Geometry: final body of the model. Coordinates: model frame, mm. A direction names the side the tool comes from. Round coordinates to 2 decimals unless told otherwise and drop trailing zeros. Loops run counter-clockwise (first coordinate to the right, second up) from the corner with the lowest first, then second, coordinate; pieces in that order, holes last. Notation, with made-up numbers: M 45.25,3 L 69.25,3 A17 ccw 69.25,11 Z; hole C 85,68 d10. An arc over 180 degrees is marked long. Answer as a JSON object with one key per item and string values.
from build123d import *

# Parameters (mm, degrees)
SKETCH2_W             = 10
SKETCH2_H             = 101.6
BOSS_EXTRUDE1_DEPTH   = 80
BOSS_EXTRUDE1_2_DEPTH = 80
SKETCH2_3_W           = 10
SKETCH2_3_H           = 101.6
SKETCH2_3_W_2         = 80
BOSS_EXTRUDE2_DEPTH   = 5
SKETCH3_R             = 14.2875
CUT_EXTRUDE1_DEPTH    = 117
SKETCH4_W             = 25.345740838
SKETCH4_H             = 80
CUT_EXTRUDE2_DEPTH    = 119
FILLET3_R             = 10
FILLET2_R             = 10
SKETCH7_R             = 1.6
CUT_EXTRUDE4_DEPTH    = 21
BOSS_EXTRUDE3_START   = 80
SKETCH8_R             = 14.2875
SKETCH8_R_2           = 7.62
BOSS_EXTRUDE3_DEPTH   = 3
SKETCH9_R             = 2.1
CUT_EXTRUDE5_DEPTH    = 5
CUT_EXTRUDE6_DEPTH    = 10
SKETCH10_R            = 2.54
CUT_EXTRUDE7_DEPTH    = 10
FILLET4_R             = 25


with BuildPart() as part:
    # Sketch2 → Boss-Extrude1 (new body)
    with BuildSketch(Plane(origin=(0, 0, 0), x_dir=(1, 0, 0), z_dir=(0, 1, 0))):
        with Locations((-45, 0)):
            Rectangle(SKETCH2_W, SKETCH2_H)
    extrude(amount=BOSS_EXTRUDE1_DEPTH)



with BuildPart() as body_2:
    # Sketch2 → Boss-Extrude1 2 (new body)
    with BuildSketch(Plane(origin=(0, 0, 0), x_dir=(1, 0, 0), z_dir=(0, 1, 0))):
        with Locations((45, 0)):
            Rectangle(SKETCH2_W, SKETCH2_H)
    extrude(amount=BOSS_EXTRUDE1_2_DEPTH)


with BuildPart() as part_1:
    add(part.part)

    add(body_2.part)  # Boss-Extrude2 merges body 2
    # Sketch2<3> → Boss-Extrude2 (add)
    with BuildSketch(Plane(origin=(0, 0, 0), x_dir=(1, 0, 0), z_dir=(0, 1, 0))):
        with Locations((45, 0)):
            Rectangle(SKETCH2_3_W, SKETCH2_3_H)
        Rectangle(SKETCH2_3_W_2, SKETCH2_3_H)
        with Locations((-45, 0)):
            Rectangle(SKETCH2_3_W, SKETCH2_3_H)
    extrude(amount=-BOSS_EXTRUDE2_DEPTH)

    # Sketch3 → Cut-Extrude1 (cut)
    with BuildSketch(Plane.ZY.offset(50)):
        with Locations((0, 50)):
            Circle(SKETCH3_R)
    extrude(amount=-CUT_EXTRUDE1_DEPTH, mode=Mode.SUBTRACT)

    # Sketch4 → Cut-Extrude2 (cut)
    with BuildSketch(Plane(origin=(50, 0, 0), x_dir=(0, 0, -1), z_dir=(1, 0, 0))):
        with Locations((-38.127129581, 40)):
            Rectangle(SKETCH4_W, SKETCH4_H)
        with Locations((38.127129581, 40)):
            Rectangle(SKETCH4_W, SKETCH4_H)
    extrude(amount=-CUT_EXTRUDE2_DEPTH, mode=Mode.SUBTRACT)

    # Fillet3
    fillet3_edges = [part_1.edges().sort_by_distance(p)[0] for p in [
        (45, 80, -25.454259162),
        (45, 80, 25.454259162),
        (40, 0, 0),
        (-40, 0, 0),
        (-45, 0, 25.454259162),
        (45, 0, 25.454259162),
        (-45, 0, -25.454259162),
        (45, 0, -25.454259162),
    ]]
    fillet(fillet3_edges, radius=FILLET3_R)

    # Fillet2
    fillet2_edges = [part_1.edges().sort_by_distance(p)[0] for p in [
        (50, -2.5, -50.8),
        (50, -2.5, 50.8),
        (-50, -2.5, 50.8),
        (-50, -2.5, -50.8),
    ]]
    fillet(fillet2_edges, radius=FILLET2_R)

    # Sketch7 → Cut-Extrude4 (cut)
    with BuildSketch(Plane(origin=(50, 0, 0), x_dir=(0, 0, -1), z_dir=(1, 0, 0))):
        with Locations((-15.5, 65.5)):
            Circle(SKETCH7_R)
        with Locations((15.5, 65.5)):
            Circle(SKETCH7_R)
        with Locations((15.5, 34.5)):
            Circle(SKETCH7_R)
        with Locations((-15.5, 34.5)):
            Circle(SKETCH7_R)
    extrude(amount=-CUT_EXTRUDE4_DEPTH, mode=Mode.SUBTRACT)

    # Sketch8 → Boss-Extrude3 (add)
    with BuildSketch(Plane.ZY.offset(-40).offset(BOSS_EXTRUDE3_START)):
        with Locations((0, 50)):
            Circle(SKETCH8_R)
        with Locations((0, 50)):
            Circle(SKETCH8_R_2, mode=Mode.SUBTRACT)
    extrude(amount=BOSS_EXTRUDE3_DEPTH)

    # Sketch9 → Cut-Extrude5 (cut)
    with BuildSketch(Plane.XZ.offset(5)):
        with Locations((-40.66, 40.66)):
            Circle(SKETCH9_R)
        with Locations((40.66, 40.66)):
            Circle(SKETCH9_R)
        with Locations((-40.66, -40.66)):
            Circle(SKETCH9_R)
        with Locations((40.66, -40.66)):
            Circle(SKETCH9_R)
    extrude(amount=-CUT_EXTRUDE5_DEPTH, mode=Mode.SUBTRACT)

    # Sketch5 → Cut-Extrude6 (cut)
    with BuildSketch(Plane(origin=(0, 0, 0), x_dir=(1, 0, 0), z_dir=(0, 1, 0))):
        with BuildLine():
            Line((-1.917657947, 2.032), (1.917657947, 2.032))
            ThreePointArc((1.917657947, 2.032), (0, -2.794), (-1.917657947, 2.032))
        make_face()
    extrude(amount=-CUT_EXTRUDE6_DEPTH, mode=Mode.SUBTRACT)

    # Sketch10 → Cut-Extrude7 (cut)
    with BuildSketch(Plane(origin=(0, 0, 0), x_dir=(1, 0, 0), z_dir=(0, 1, 0))):
        with Locations((0, 9.099794366)):
            Circle(SKETCH10_R)
    extrude(amount=-CUT_EXTRUDE7_DEPTH, mode=Mode.SUBTRACT)

    # Fillet4
    fillet4_edges = [part_1.edges().sort_by_distance(p)[0] for p in [
        (-45, 80, 25.454259162),
        (-45, 80, -25.454259162),
    ]]
    fillet(fillet4_edges, radius=FILLET4_R)


solid = part_1.part
1) Section query B-B (y = 15). Return the cut outline in (x, z).
Results:
{"outline": "M -50,-25.45 L -40,-25.45 L -40,25.45 L -50,25.45 Z; M 40,-25.45 L 50,-25.45 L 50,25.45 L 40,25.45 Z"}
2) Section query D-D (z = -30.5). Return the cut outline in (x, y), and give its area (3 significant figures).
Results:
{"outline": "M -50,-5 L 50,-5 L 50,1.31 L 34.95,1.31 A10 cw 30,0 L -30,0 A10 cw -34.95,1.31 L -50,1.31 Z", "area": "544 mm2"}
3) Section query A-A (y = 50). Return the cut outline in (x, z).
Results:
{"outline": "M -50,-25.45 L -40,-25.45 L -40,-7.62 L -43,-7.62 L -43,-14.29 L -50,-14.29 Z; M -50,14.29 L -43,14.29 L -43,7.62 L -40,7.62 L -40,25.45 L -50,25.45 Z; M 40,-25.45 L 50,-25.45 L 50,-14.29 L 40,-14.29 Z; M 40,14.29 L 50,14.29 L 50,25.45 L 40,25.45 Z"}
4) Section query C-C (x = -37). Return the cut outline in (y, z), and give its area (3 significant figures).
Results:
{"outline": "M -5,-50.8 L 0,-50.8 L 0,-35.45 A10 cw 2.86,-28.45 L 2.86,28.45 A10 cw 0,35.45 L 0,50.8 L -5,50.8 Z", "area": "683 mm2"}
5) Ray query, line 1 (Y direction, x = 45.75, z = 15.5); line 2 (X direction, y = 17, z = 8.5); line 3 (Y direction, x = -47, z = 0). Return the intervals inside material, ascending.
Results:
{"line 1": "-5 to 32.9, 36.1 to 63.9, 67.1 to 80", "line 2": "-50 to -40, 40 to 50", "line 3": "-5 to 35.71, 64.29 to 80"}
6) Reachability of faces 1 (the flat face through (40, 36.7, 6)), 2 (the cylindrical face through (-46.549, 36.052, -3.097)), 3 (the flat face through (-45, 32, -25.454)) from +Z, -Z, +X, -X, +Y, -Y: full face, straight path, thin tool, end or side. Return the list, or none.
Results:
{"face 1": "+Z, -Z, +Y", "face 2": "-X", "face 3": "-Z, +X, -X, +Y"}
7) Pull-direction query (Y, two-part tool) for faces 4 (the flat face through (-43, 44, 6)), 5 (the cylindrical face through (-42.36, 1.87, 29.63)), 6 (the flat face through (-1, -2, 50.8)); classes: +Y half, -Y half, draft (parallel to the pull), parting line (faces both ways), or undercut.
Results:
{"face 4": "undercut", "face 5": "+Y half", "face 6": "draft"}
8) Pin query (flat end, axial travel): P1, Ø4, axis at x = -32, z = 2, coming from the +Y side; P2, Ø6.5, axis at x = 0, z = 0, coming from the +Y side; P3, Ø3, axis at y = 34.5, z = -15.5, coming from the +X side; P4, Ø3.5, axis at x = -40.66, z = -40.66, coming from the +Y side. Return the tip coordinate at first contact, or that it passes through.
Results:
{"P1": "y = 0.83", "P2": "y = 0", "P3": "x = -40", "P4": "through"}
